Geometry check sheet. Reference: the model listing, model coordinates, mm. Face numbers are marked on the shaded views. A direction names the side the tool comes from. Round coordinates to 2 decimals unless told otherwise and drop trailing zeros. Order: outer loops, then holes, each group sorted by start corner. A loop starts at its lowest first (then second) coordinate and runs counter-clockwise, first axis right, second up.
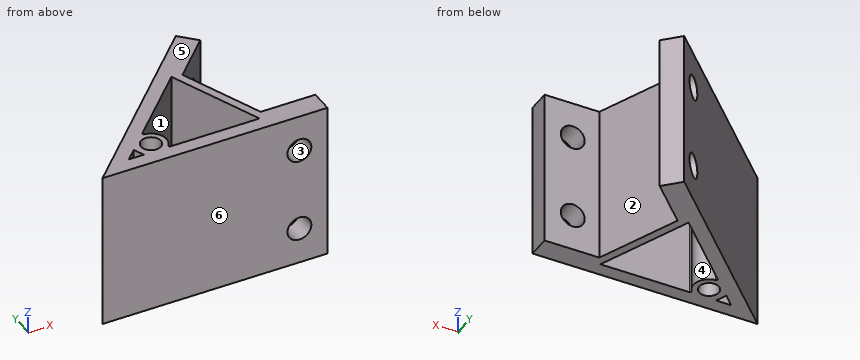
```python
from build123d import *

# Parameters (mm, degrees)
SKETCH_1_R          = 3.5
EXTRUDE_1_DEPTH     = 28
SKETCH_3_R          = 4.25
CUT_EXTRUDE_2_DEPTH = 20


with BuildPart() as part:
    # 草图1 → 凸台-拉伸1 (new, symmetric)
    with BuildSketch(Plane.XY):
        Polygon((0, 0), (56.568542495, 56.568542495), (62.225396744, 50.911688245), (48.470353518, 37.156645019), (60.547431318, 8), (80, 8), (80, 0), align=None)
        with Locations((22.184677187, 9.156473773)):
            Circle(SKETCH_1_R, mode=Mode.SUBTRACT)
        Polygon((12.071067812, 5), (15.847671377, 8.776603565), (17.411991793, 5), align=None, mode=Mode.SUBTRACT)
        with BuildLine():
            Line((22.539170943, 15.468103131), (44.931612237, 37.860544425))
            Line((44.931612237, 37.860544425), (58.542895405, 5))
            Line((58.542895405, 5), (26.941798117, 5))
            ThreePointArc((26.941798117, 5), (26.493271042, 5.27903968), (26.545371373, 5.804706148))
            ThreePointArc((26.545371373, 5.804706148), (27.253512915, 11.291164467), (22.833720405, 14.61804341))
            ThreePointArc((22.833720405, 14.61804341), (22.420282519, 14.950846558), (22.539170943, 15.468103131))
        make_face(mode=Mode.SUBTRACT)
    extrude(amount=EXTRUDE_1_DEPTH, both=True)

    # 草图3 → 切除-拉伸2 (cut)
    with BuildSketch(Plane.XZ):
        with Locations(Location((70, 15, 0), (0, 0, 270))):
            Circle(SKETCH_3_R)
        with Locations(Location((70, -15, 0), (0, 0, 270))):
            Circle(SKETCH_3_R)
    cut_extrude_2 = extrude(amount=-CUT_EXTRUDE_2_DEPTH, mode=Mode.SUBTRACT)

    # 镜向1: 切除-拉伸2 across plane
    add(cut_extrude_2.mirror(Plane(origin=(0, 0, 0), x_dir=(0, 0, 1), z_dir=(0.3826834323650904, -0.9238795325112865, 0))), mode=Mode.SUBTRACT)


solid = part.part
```
(1) Set-up check for the marked faces 1, 2 and 3: record each of +Z, -Z, +X, -X, +Y, -Y from which the full face is reachable in a straight line by a thin tool's end or side.
Returned:
face 1: +Z, -Z
face 2: +Z, -Z, +X
face 3: +Y, -Y
(2) Sectioned sample at C-C, the plane y = 17. Record the cut outline in (x, z), and give its area (3 significant figures).
Returned:
outline: (17, -28) - (24.07, -28) - (24.07, 28) - (17, 28) - close; (53.57, -28) - (56.82, -28) - (56.82, 28) - (53.57, 28) - close
area: 578 mm2
(3) Sectioned sample at B-B, the plane x = 70. Record the cut outline in (y, z), and give its area (3 significant figures).
Returned:
outline: (0, -28) - (8, -28) - (8, -19.25) - (0, -19.25) - close; (0, -10.75) - (8, -10.75) - (8, 10.75) - (0, 10.75) - close; (0, 19.25) - (8, 19.25) - (8, 28) - (0, 28) - close
area: 312 mm2
(4) Draft check along Y on the marked faces 4, 5 and 6. Enter one of: released by +Y, released by -Y, zero draft, split by the parting line, or undercut.
Returned:
face 4: undercut
face 5: zero draft
face 6: released by -Y
(5) Sectioned sample at A-A, the plane z = 15. Record the cut outline in (x, y).
Returned:
outline: (0, 0) - (65.75, 0) - (65.75, 8) - (60.55, 8) - (48.47, 37.16) - (52.15, 40.84) - (46.49, 46.49) - close; (52.5, 52.5) - (58.16, 46.85) - (62.23, 50.91) - (56.57, 56.57) - close; (74.25, 0) - (80, 0) - (80, 8) - (74.25, 8) - close; hole (12.07, 5) - (17.41, 5) - (15.85, 8.78) - close; hole circle Ø7 at (22.18, 9.16); hole (22.54, 15.47) arc R0.5 ccw to (22.83, 14.62) arc R5.5 cw to (26.55, 5.8) arc R0.5 ccw to (26.94, 5) - (58.54, 5) - (44.93, 37.86) - close
(6) Depth check by flat-ended pin: P1, Ø1.5, axis at y = 31.5, z = 1, coming from the +X side; P2, Ø4.5, axis at x = 15, z = 6, coming from the +Y side; P3, Ø4, axis at x = 31, z = 17.5, coming from the +Y side. Enter the tip coordinate at first touch or a pass-through.
Returned:
P1: stops at x = 51.12
P2: stops at y = 17.25
P3: stops at y = 33
(7) Material ranges on line 1 (Y direction, x = 55.5, z = 20); line 2 (X direction, y = 6, z = 15); line 3 (Y direction, x = 74, z = -11.5), recorded low to high.
Returned:
line 1: y = 0 to 5, 12.35 to 20.19, 44.19 to 55.5
line 2: x = 6 to 13.07, 17 to 20.67, 23.7 to 26.69, 58.13 to 65.75, 74.25 to 80
line 3: y = 0 to 8
(8) Sectioned sample at D-D, the plane y = 4. Record the cut outline in (x, z).
Returned:
outline: (4, -28) - (80, -28) - (80, 28) - (4, 28) - close; hole circle Ø8.5 at (70, -15); hole circle Ø8.5 at (70, 15)
